Input: part model. Units: mm. Frame: model coordinates. Coordinates: 2 decimals unless noted, no trailing zeros. Loops run counter-clockwise (first coordinate to the right, second up) from the corner with the lowest first, then second, coordinate; pieces in that order, holes last. Notation, with made-up numbers: (30, 10.5) - (80, 10.5) arc R6 ccw to (80, 19.5) - close; hole circle Ø3 at (-27.5, 19.25). An arc over 180 degrees is marked (long way). Use a Markdown table: item, result. Add a question column.
1. Draft query along Z for faces 1 (the face through (4, 0, 6)), 2 (the face through (0, -4, 2)), 3 (the face through (3.948, -3.905, 0.867)). Return one class per face: released by +Z, released by -Z, zero draft, split by the parting line, or undercut.
2. Section query C-C on x = 0.5. Return the cut outline in (y, z).
3. Ray query, L1, parallel to Y at x = 6, z = 0; L2, parallel to Y at x = 4.5, z = 1.25; L3, parallel to Z at x = 7.25, y = 1.75. Return the intervals inside material, ascending. Write a range as [from, to].
4. Contact query for flat-ended pins moving along their axis: P1, Ø6, axis at y = 2.5, z = 2.5, coming from the +X side; P2, Ø1, axis at x = 1, z = -3.5, coming from the -Y side; P3, Ø2, axis at x = 1.5, z = -1.5, coming from the -Y side; P4, Ø2, axis at x = 3, y = 3, coming from the -Z side. Output: stop coordinate, or through.
5. Section query A-A on y = 0. Return the cut outline in (x, z), then the cut area to 4 significant figures.
```python
from build123d import *

# Parameters (mm, degrees)
SKETCH1_R           = 6
SKETCH1_R_2         = 4
BOSS_EXTRUDE1_DEPTH = 8
CHAMFER1_SIZE       = 0.25


with BuildPart() as part:
    # Sketch1 → Boss-Extrude1 (new body)
    with BuildSketch(Plane(origin=(0, 0, 0), x_dir=(0, 0, -1), z_dir=(1, 0, 0))):
        Circle(SKETCH1_R)
        Circle(SKETCH1_R_2, mode=Mode.SUBTRACT)
    extrude(amount=BOSS_EXTRUDE1_DEPTH)

    # Chamfer1
    chamfer1_edges = [part.edges().sort_by_distance(p)[0] for p in [
        (0, 0, 6),
        (8, 0, 6),
        (0, 0, 4),
        (8, 0, 4),
    ]]
    chamfer(chamfer1_edges, length=CHAMFER1_SIZE)


solid = part.part
```
Resolved:
| question | item | result |
|---|---|---|
| 1 | face 1 | split by the parting line |
| 1 | face 2 | zero draft |
| 1 | face 3 | undercut |
| 2 | outline | circle Ø12 at (0, 0); hole circle Ø8 at (0, 0) |
| 3 | L1 | [-6, -4], [4, 6] |
| 3 | L2 | [-5.87, -3.8], [3.8, 5.87] |
| 3 | L3 | [-5.74, -3.6], [3.6, 5.74] |
| 4 | P1 | x = 8 |
| 4 | P2 | y = -5.2 |
| 4 | P3 | y = -5.98 |
| 4 | P4 | z = -5.66 |
| 5 | outline | (0, -5.75) - (0.25, -6) - (7.75, -6) - (8, -5.75) - (8, -4.25) - (7.75, -4) - (0.25, -4) - (0, -4.25) - close; (0, 4.25) - (0.25, 4) - (7.75, 4) - (8, 4.25) - (8, 5.75) - (7.75, 6) - (0.25, 6) - (0, 5.75) - close |
| 5 | area | 31.75 mm² |
